Can you work these out from the model? Positions are in its coordinate system, mm. A direction names the side the tool comes from. Coordinates: 2 decimals unless noted, no trailing zeros. Order: outer loops, then holes, each group sorted by start corner. A loop starts at its lowest first (then second) coordinate and runs counter-clockwise, first axis right, second up.
Autodesk Inventor part; units mm, degrees
ref_plane "YZ Plane" through (0, 0, 0) normal (1, 0, 0) x (0, 1, 0)
ref_plane "XZ Plane" through (0, 0, 0) normal (0, 1, 0) x (-1, 0, 0)
ref_plane "XY Plane" through (0, 0, 0) normal (0, 0, 1) x (1, 0, 0)
sketch "Sketch1" plane through (0, 0, 0) normal (0, 1, 0) x (-1, 0, 0)
  line L0 (174.625, 74.6125) -> (-174.625, 74.6125)
  line L1 (-174.625, 74.6125) -> (-174.625, -74.6125)
  line L2 (-174.625, -74.6125) -> (174.625, -74.6125)
  line L3 (174.625, -74.6125) -> (174.625, 74.6125)
  line L4 (174.625, 74.6125) -> (-174.625, -74.6125) construction
  line L5 (-174.625, 74.6125) -> (174.625, -74.6125) construction
  point P0 (0, 0)
  dimension "d0" = 149.225
  dimension "d4" = 349.25
extrude "Extrusion1" add sketch "Sketch1" against normal blind 19.05
sketch "Sketch3" plane through (-174.625, 0, 74.6125) normal (0, 0, 1) x (1, 0, 0)
  line L0 (0, 0) -> (349.25, 0)
  line L1 (0, 0) -> (0, -19.05)
  line L2 (349.25, 0) -> (349.25, -19.05)
  line L3 (0, 0) -> (349.25, 0)
  line L4 (349.25, 0) -> (349.25, -228.6)
  line L5 (349.25, -228.6) -> (0, -228.6)
  line L6 (0, -228.6) -> (0, 0)
  point P0 (174.625, 0)
  dimension "d5" = 228.6
extrude "Extrusion2" add sketch "Sketch3" along normal blind 19.05
mirror "Mirror1" about plane through (0, 0, 0) normal (0, 0, 1) of "Extrusion2"
sketch "Sketch4" plane through (-174.625, 0, 93.6625) normal (0, 0, 1) x (1, 0, 0)
  line L0 (174.625, 0) -> (174.625, -228.6) construction
  line L1 (0, -228.6) -> (349.25, -228.6) construction
  point P0 (174.625, -207.6224)
hole "Hole1" at (0, -207.6224, 93.6625) direction (0, 0, -1) diameter 6.7564 end through all
pattern_linear "Rectangular Pattern1" count 4 spacing 25.4 along (0, 1, 0) of "Hole1"
sketch "Sketch5" plane through (0, 0, 0) normal (0, 1, 0) x (1, 0, 0)
  circle A0 centre (0, 0) radius 63.5
  dimension "d18" = 127
extrude "Extrusion3" cut sketch "Sketch5" against normal blind 2.54
equation "\"d0\" = widthTopBoard"
equation "\"d4\" = lengthTopBoard"
equation "\"d1\" = woodThickness"
equation "\"d6\" = woodThickness"
equation "\"widthTopBoard\" = 149.225"
equation "\"lengthTopBoard\" = 349.25"
equation "\"woodThickness\" = 19.05"
properties part number "woodBracketForCamera" material "Wood (Birch)"
1. Imagine slicing it at A-A on y = -44. Please give me the cut outline in (x, z) (1 decimal).
Completed:
outline: (-174.6, -93.7) - (174.6, -93.7) - (174.6, -74.6) - (-174.6, -74.6) - close; (-174.6, 74.6) - (174.6, 74.6) - (174.6, 93.7) - (-174.6, 93.7) - close
2. Imagine slicing it at C-C on z = 8.5. Please give me the cut outline in (x, y) (3 decimals), then the cut area to 3 significant figures.
Completed:
outline: (-174.625, -19.05) - (174.625, -19.05) - (174.625, 0) - (62.929, 0) - (62.929, -2.54) - (-62.929, -2.54) - (-62.929, 0) - (-174.625, 0) - close
area: 6,330 mm2
3. Imagine slicing it at B-B on x = -121. Please give me the cut outline in (y, z).
Completed:
outline: (-228.6, -93.66) - (0, -93.66) - (0, 93.66) - (-228.6, 93.66) - (-228.6, 74.61) - (-19.05, 74.61) - (-19.05, -74.61) - (-228.6, -74.61) - close
4. Please list where these lines run through material, in increasing order: probe 1 along Y at (x, z) = (0, 87); probe 2 along Z at (x, y) = (-139.5, -99); probe 3 along Y at (x, z) = (-60, 33.5).
Completed:
probe 1: y = -228.6 to -211, -204.24 to -185.6, -178.84 to -160.2, -153.44 to -134.8, -128.04 to 0
probe 2: z = -93.66 to -74.61, 74.61 to 93.66
probe 3: y = -19.05 to 0
5. On a 3-axis mill with a long thin cutter (end or side, diameter ignored), from which of +Z, -Z, +X, -X, +Y, -Y can I reach the whole of each face in a straight line? I mean faces 1 (the flat face through (2, -228.6, 84)), 2 (the flat face through (2, -19.05, 1)), 3 (the cylindrical face through (-13.77, -1.25, 61.99)). Say none if no direction works.
Completed:
face 1: +Z, -Z, +X, -X, -Y
face 2: +X, -X, -Y
face 3: +Y
6. Thinking about a two-plate mould opening in X: for faces 4 (the flat face through (2, 0, 64)), 5 (the flat face through (174.625, -89, -76)), 6 (the flat face through (-1, -2.54, -1)), which applies, pulls with the +X half, pulls with the -X half, needs draft (parallel to the pull), parting line crosses it, or undercut?
Completed:
face 4: needs draft
face 5: pulls with the +X half
face 6: undercut
7. I'm going to push flat-ended pins straight in: pin 1 (4 mm diameter, centred on x = 0, y = -182.22, fed in from +Z); pin 2 (1.5 mm diameter, centred on x = -5.5, z = 45.5, fed in from +Y); pin 3 (1 mm diameter, centred on x = 105, z = 26, fed in from -Y). Where does each tip first touch, or does it pass through?
Completed:
pin 1: passes through
pin 2: stops at y = -2.54
pin 3: stops at y = -19.05
8. Imagine slicing it at D-D on x = -22. Please give me the cut outline in (y, z).
Completed:
outline: (-228.6, -93.66) - (0, -93.66) - (0, -59.57) - (-2.54, -59.57) - (-2.54, 59.57) - (0, 59.57) - (0, 93.66) - (-228.6, 93.66) - (-228.6, 74.61) - (-19.05, 74.61) - (-19.05, -74.61) - (-228.6, -74.61) - close
